CAD build for the part. Positions are in the model's coordinates, mm. Face numbers are marked on the shaded views. A direction names the side the tool comes from. Give positions to 0.01 mm unless a question says otherwise; leave off trailing zeros. Write each loop counter-clockwise with the first axis right and the second up, starting at its lowest first coordinate (ties: lowest second). Pieces come first, ordered by that corner, then holes. Notation, with made-up numbers: M -32.75,33.5 L 4.25,33.5 A30 ccw 4.25,62.5 Z; hole C 0.5,-38 d1. An arc over 180 degrees is marked long. One line per question, with ' | ' between items. Start each with the question number.
1. Cut at D-D, the plane x = 20. Write the cut outline in (y, z).
2. Which spindle directions (+Z, -Z, +X, -X, +Y, -Y) get a long thin tool onto all of the face, cutting with end or side? Do the marked faces 4 and 5. Say none if no direction does.
3. Cut at A-A, the plane x = -7.5. Write the cut outline in (y, z), then the cut area to 3 significant figures.
4. Wall check: L1, parallel to X at y = -2, z = 1.75; L2, parallel to X at y = -10.5, z = 5.25; L3, parallel to Y at x = -7.5, z = 3.75. Give the ranges that are in metal, low to high.
5. Cut at B-B, the plane z = 12.25. Write the cut outline in (x, y), then the cut area to 3 significant figures.
6. Cut at C-C, the plane y = -11.5. Write the cut outline in (x, z).
7. Pull direction X, two halves, no side cores. Call the marked faces 1, 2 and 3: released by +X, released by -X, zero draft, split by the parting line, or undercut.
8. Flat gauge pins, fed straight in: pin 1 (2 mm diameter, centred on y = -7.5, z = 12.5, fed in from -X); pin 2 (4 mm diameter, centred on y = 5.5, z = 8.5, fed in from -X); pin 3 (3 mm diameter, centred on y = 0, z = 6.5, fed in from -X). Where does each tip first touch, or does it go through?
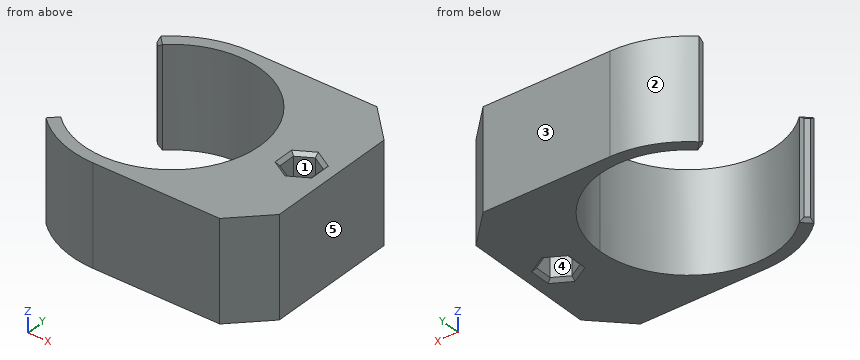
```python
from build123d import *

# Parameters (mm, degrees)
F1_DEPTH    = 15
F2_T1_DEPTH = 17.6582428067
F2_T3_DEPTH = 17.5274686085
F2_T5_DEPTH = 4.321682988
F2_T7_DEPTH = 4.321682988
F3_SIZE     = 5
F4_SIZE     = 0.5


# Not quite as in the source:
# - a fillet or chamfer that OpenCascade refuses, or shapes differently, is made with other operations: its cross-section is extruded or revolved along the edge and cut away or added


with BuildPart() as f1:
    # F0 (on Top) → F1 (new body)
    with BuildSketch(Plane.XY):
        with BuildLine():
            ThreePointArc((0, -15), (10.6066017178, -10.6066017178), (15, 0))
            ThreePointArc((15, 0), (10.6066017178, 10.6066017178), (0, 15))
            ThreePointArc((0, 15), (-5.7402514855, 13.8581929877), (-10.6066017178, 10.6066017178))
            Line((-10.6066017178, 10.6066017178), (-9.3691648507, 9.3691648507))
            ThreePointArc((-9.3691648507, 9.3691648507), (5.0705554788, 12.2414038058), (13.25, 0))
            ThreePointArc((13.25, 0), (5.0705554788, -12.2414038058), (-9.3691648507, -9.3691648507))
            Line((-9.3691648507, -9.3691648507), (-10.6066017178, -10.6066017178))
            ThreePointArc((-10.6066017178, -10.6066017178), (-5.7402514855, -13.8581929877), (0, -15))
        make_face()
        with BuildLine():
            ThreePointArc((0, 15), (10.6066017178, 10.6066017178), (15, 0))
            ThreePointArc((15, 0), (10.6066017178, -10.6066017178), (0, -15))
            Line((0, -15), (24, -15))
            Line((24, -15), (24, 15))
            Line((24, 15), (0, 15))
        make_face()
        Polygon((19.5, -2.5980762114), (17.25, -1.2990381057), (17.25, 1.2990381057), (19.5, 2.5980762114), (21.75, 1.2990381057), (21.75, -1.2990381057), align=None, mode=Mode.SUBTRACT)
    extrude(amount=F1_DEPTH)

    # F2: chamfer of 0.5 on 8 edges, made by hand

    # F2_s2 → F2_t1 (cut)
    with BuildSketch(Plane.XY.offset(-1.3291214034)):
        with BuildLine():
            Line((-10.234549009, 10.9660387826), (-10.246950766, 10.246950766))
            Line((-10.246950766, 10.246950766), (-10.6066017178, 10.6066017178))
            ThreePointArc((-10.6066017178, 10.6066017178), (-10.4170400144, 10.7928345368), (-10.234549009, 10.9660387826))
        make_face()
        with BuildLine():
            Line((-10.246950766, -10.246950766), (-10.234549009, -10.9660387826))
            ThreePointArc((-10.234549009, -10.9660387826), (-10.4170400144, -10.7928345368), (-10.6066017178, -10.6066017178))
            Line((-10.6066017178, -10.6066017178), (-10.246950766, -10.246950766))
        make_face()
    extrude(amount=F2_T1_DEPTH, mode=Mode.SUBTRACT)

    # F2_s4 → F2_t3 (cut)
    with BuildSketch(Plane.XY.offset(-1.2637343043)):
        with BuildLine():
            Line((-9.7162878714, 9.7162878714), (-9.0222714088, 9.7036652161))
            ThreePointArc((-9.0222714088, 9.7036652161), (-9.1921439944, 9.5429025346), (-9.3691648507, 9.3691648507))
            Line((-9.3691648507, 9.3691648507), (-9.7162878714, 9.7162878714))
        make_face()
        with BuildLine():
            Line((-9.7162878714, -9.7162878714), (-9.0222714088, -9.7036652161))
            ThreePointArc((-9.0222714088, -9.7036652161), (-9.1921439944, -9.5429025346), (-9.3691648507, -9.3691648507))
            Line((-9.3691648507, -9.3691648507), (-9.7162878714, -9.7162878714))
        make_face()
    extrude(amount=F2_T3_DEPTH, mode=Mode.SUBTRACT)

    # F2_s6 → F2_t5 (cut)
    with BuildSketch(Plane(origin=(-11.5158289577, 11.5158289577, 0), x_dir=(0, 0, 1), z_dir=(0.7071067812, -0.7071067812, 0))):
        Polygon((0.5, 0), (0, -0.5), (0, 0), align=None)
        Polygon((14.5, 0), (15, -0.5), (15, 0), align=None)
    extrude(amount=F2_T5_DEPTH, mode=Mode.SUBTRACT)

    # F2_s8 → F2_t7 (cut)
    with BuildSketch(Plane(origin=(-8.4599376108, -8.4599376108, 0), x_dir=(0, 0, 1), z_dir=(-0.7071067812, -0.7071067812, 0))):
        Polygon((0.5, 0), (0, -0.5), (0, 0), align=None)
        Polygon((14.5, 0), (15, -0.5), (15, 0), align=None)
    extrude(amount=F2_T7_DEPTH, mode=Mode.SUBTRACT)

    # F3
    f3_edges = [f1.edges().sort_by_distance(p)[0] for p in [
        (24, -15, 7.5),
        (24, 15, 7.5),
    ]]
    chamfer(f3_edges, length=F3_SIZE)

    # F4
    f4_edges = [f1.edges().sort_by_distance(p)[0] for p in [
        (18.375, 1.948557, 15),
        (20.625, 1.948557, 15),
        (21.75, 0, 15),
        (20.625, -1.948557, 15),
        (18.375, -1.948557, 15),
        (17.25, 0, 15),
        (20.625, 1.948557, 0),
        (21.75, 0, 0),
        (20.625, -1.948557, 0),
        (18.375, -1.948557, 0),
        (17.25, 0, 0),
        (18.375, 1.948557, 0),
    ]]
    chamfer(f4_edges, length=F4_SIZE)


solid = f1.part
```
Here are the results:
1) outline: M -14,0 L -2.89,0 L -2.31,0.5 L -2.31,14.5 L -2.89,15 L -14,15 Z; M 2.31,0.5 L 2.89,0 L 14,0 L 14,15 L 2.89,15 L 2.31,14.5 Z
2) face 4: +Z, -Z | face 5: +Z, -Z, +X, +Y, -Y
3) outline: M -12.99,0 L -10.92,0 L -10.92,15 L -12.99,15 Z; M 10.92,0 L 12.99,0 L 12.99,15 L 10.92,15 Z | area: 62.0 mm^2
4) L1: 13.1 to 18.46, 20.54 to 24 | L2: -10.24 to -8.08, 8.08 to 23.5 | L3: -12.99 to -10.92, 10.92 to 12.99
5) outline: M -10.25,-10.25 L -10.23,-10.97 A15 ccw 0,-15 L 19,-15 L 24,-10 L 24,10 L 19,15 L 0,15 A15 ccw -10.23,10.97 L -10.25,10.25 L -9.72,9.72 L -9.02,9.7 A13.25 cw long -9.02,-9.7 L -9.72,-9.72 Z; hole M 17.25,-1.3 L 19.5,-2.6 L 21.75,-1.3 L 21.75,1.3 L 19.5,2.6 L 17.25,1.3 Z | area: 440 mm^2
6) outline: M -9.63,0 L -6.58,0 L -6.58,15 L -9.63,15 Z; M 6.58,0 L 22.5,0 L 22.5,15 L 6.58,15 Z
7) face 1: undercut | face 2: released by -X | face 3: zero draft
8) pin 1: x = 10.16 | pin 2: x = 10.92 | pin 3: x = 13.16
